Check sheet for the modelled part. Datum: model origin and axes. Units: mm. Round coordinates to 2 decimals unless told otherwise and drop trailing zeros. Order: outer loops, then holes, each group sorted by start corner. A loop starts at its lowest first (then second) coordinate and runs counter-clockwise, first axis right, second up. Notation, with made-up numbers: (-38.75, -3.5) -> (-34.75, -3.5) arc R26 cw to (-34.75, 14.5) -> close; hole circle Ø11 at (-16, 68.25). An arc over 180 degrees is marked (long way). Answer in a Markdown table with one row per item.
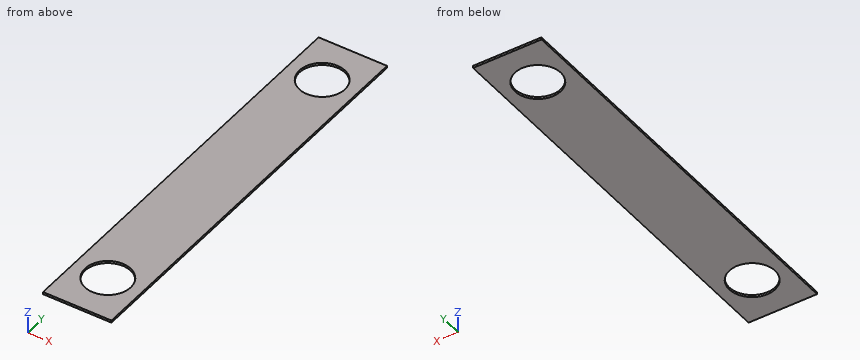
Autodesk Inventor part; units mm, degrees
ref_plane "YZ Plane" through (0, 0, 0) normal (1, 0, 0) x (0, 1, 0)
ref_plane "XZ Plane" through (0, 0, 0) normal (0, 1, 0) x (-1, 0, 0)
ref_plane "XY Plane" through (0, 0, 0) normal (0, 0, 1) x (1, 0, 0)
sketch "Sketch1" plane through (0, 0, 0) normal (0, 0, 1) x (1, 0, 0)
  line L0 (0, 0) -> (15, 0)
  line L1 (15, 0) -> (15, -90)
  line L2 (15, -90) -> (0, -90)
  line L3 (0, -90) -> (0, 0)
  dimension "d0" = 15
  dimension "d1" = 90
extrude "Plate1" add sketch "Sketch1" along normal blind 0.5
sketch "Sketch2" plane through (0, 0, 0.5) normal (0, 0, 1) x (1, 0, 0)
  line L0 (0, 0) -> (15, 0)
  line L1 (7.5, 0) -> (7.5, -10)
  circle A0 centre (7.5, -10) radius 5
  line L2 (15, -90) -> (0, -90)
  line L3 (7.5, -90) -> (7.5, -80)
  circle A1 centre (7.5, -80) radius 5
  dimension "d3" = 10
  dimension "d4" = 10
  dimension "d5" = 10
  dimension "d6" = 10
extrude "Extrusion1" cut sketch "Sketch2" against normal blind 10
equation "\"d2\" = Thickness"
equation "\"BendRadius\" = Thickness"
equation "\"BendReliefWidth\" = Thickness"
equation "\"BendReliefDepth\" = 0.5 * Thickness"
equation "\"CornerReliefSize\" = 4 * Thickness"
equation "\"MinimumRemnant\" = 2 * Thickness"
equation "\"TransitionRadius\" = BendRadius"
equation "\"JacobiRadiusSize\" = BendRadius"
equation "\"GapSize\" = Thickness"
properties part number "shaft for capping system"
Item 1: Cross-section at A-A (x = 7.5). Record the boundary of the cut face in (y, z), and give its area (3 significant figures).
Result sheet:
| item | result |
|---|---|
| outline | (-90, 0) -> (-85, 0) -> (-85, 0.5) -> (-90, 0.5) -> close; (-75, 0) -> (-15, 0) -> (-15, 0.5) -> (-75, 0.5) -> close; (-5, 0) -> (0, 0) -> (0, 0.5) -> (-5, 0.5) -> close |
| area | 35.0 mm^2 |
Item 2: Cross-section at C-C (z = 0.1). Record the boundary of the cut face in (x, y).
Result sheet:
| item | result |
|---|---|
| outline | (0, -90) -> (15, -90) -> (15, 0) -> (0, 0) -> close; hole circle Ø10 at (7.5, -80); hole circle Ø10 at (7.5, -10) |
Item 3: Cross-section at B-B (y = -7). Record the boundary of the cut face in (x, z).
Result sheet:
| item | result |
|---|---|
| outline | (0, 0) -> (3.5, 0) -> (3.5, 0.5) -> (0, 0.5) -> close; (11.5, 0) -> (15, 0) -> (15, 0.5) -> (11.5, 0.5) -> close |
Item 4: Scan lines: line 1 (Y direction, x = 7.5, z = 0.4); line 2 (X direction, y = -80, z = 0.35); line 3 (Y direction, x = 10.5, z = 0.3). Record each from-to range of solid material in increasing order. Write a range as [from, to].
Result sheet:
| item | result |
|---|---|
| line 1 | y = [-90, -85], [-75, -15], [-5, 0] |
| line 2 | x = [0, 2.5], [12.5, 15] |
| line 3 | y = [-90, -84], [-76, -14], [-6, 0] |
